from build123d import *

# Parameters (mm, degrees)
F0_W     = 5
F0_H     = 12
F1_DEPTH = 10
F3_D     = 5


with BuildPart() as f1:
    # F0 (on Top) → F1 (new body)
    with BuildSketch(Plane.XY):
        with Locations((2.5, 6)):
            Rectangle(F0_W, F0_H)
    extrude(amount=F1_DEPTH)

    # F3 (through all)
    with Locations(Plane.YZ.offset(5)):
        with Locations((6, 5)):
            Hole(F3_D / 2)


solid = f1.part
Geometry check sheet. Reference: the model listing, model coordinates, mm. Round coordinates to 2 decimals unless told otherwise and drop trailing zeros. Write each loop counter-clockwise with the first axis right and the second up, starting at its lowest first coordinate (ties: lowest second). Pieces come first, ordered by that corner, then holes. Notation, with made-up numbers: (21, -36.75) -> (66, -36.75) arc R23 cw to (66, -19.75) -> close; hole circle Ø9 at (35, 58.25). An arc over 180 degrees is marked (long way). One line per item, written item: value. Start each with the question number.
(1) Cross-section at C-C, the plane x = 2.5. Record the cut outline in (y, z), and give its area (3 significant figures).
(2) Cross-section at B-B, the plane y = 6. Record the cut outline in (x, z).
(3) Draft check along Y on faces 1 (the flat face through (2, 12, 5)), 2 (the cylindrical face through (2.465, 3.615, 5.751)), 3 (the flat face through (2, 6, 0)). Enter one of: +Y half, -Y half, draft (parallel to the pull), parting line (faces both ways), or undercut.
(4) Scan lines: line 1 (Z direction, x = 3.65, y = 6); line 2 (Y direction, x = 3.1, z = 3.25); line 3 (Z direction, x = 1.45, y = 5.25). Record each from-to range of solid material in increasing order. Write a range as [from, to].
(5) Cross-section at A-A, the plane z = 5. Record the cut outline in (x, y), and give its area (3 significant figures).
Answer:
1. outline: (0, 0) -> (12, 0) -> (12, 10) -> (0, 10) -> close; hole circle Ø5 at (6, 5)
1. area: 100 mm²
2. outline: (0, 0) -> (5, 0) -> (5, 2.5) -> (0, 2.5) -> close; (0, 7.5) -> (5, 7.5) -> (5, 10) -> (0, 10) -> close
3. face 1: +Y half
3. face 2: undercut
3. face 3: draft
4. line 1: [0, 2.5], [7.5, 10]
4. line 2: [0, 4.21], [7.79, 12]
4. line 3: [0, 2.62], [7.38, 10]
5. outline: (0, 0) -> (5, 0) -> (5, 3.5) -> (0, 3.5) -> close; (0, 8.5) -> (5, 8.5) -> (5, 12) -> (0, 12) -> close
5. area: 35.0 mm²
